The model under review builds one solid part; all positions refer to its coordinate system, in mm. Face numbers are marked on the shaded views. Round coordinates to 2 decimals unless told otherwise and drop trailing zeros. Order: outer loops, then holes, each group sorted by start corner. A loop starts at its lowest first (then second) coordinate and runs counter-clockwise, first axis right, second up. Notation, with made-up numbers: M 22,-38.75 L 58,-38.75 A8 ccw 58,-29.75 Z; hole C 83,51 d5. An arc over 180 degrees is marked long. Answer as a JSON object with one key per item and string values. Group by question number.
1. Mouldability with a two-part tool opening along X and no side actions: class the marked faces 1 and 2 as released by +X, released by -X, zero draft, split by the parting line, or undercut.
2. Add section D-D on x = 319. State the section outline as (y, z) points.
3. To check wall thickness, follow probe 1 along X at (y, z) = (-7.5, -1.5); probe 2 along X at (y, z) = (13, 0.5) (3 decimals); probe 3 along Z at (x, y) = (396, -4). State the ranges of each line that lie inside material, in increasing order. Write a range as [from, to].
4. Add section A-A on x = 400. State the section outline as (y, z) points, and give its area (3 significant figures).
5. Add section C-C on y = -6.5. State the section outline as (x, z) points.
6. Clearance check with flat-ended pins moving along their axes: P1, Ø10, axis at y = 11.5, z = 22.5, coming from the -X side; P2, Ø1, axis at x = 301.5, y = -3, coming from the -Z side; P3, Ø8, axis at y = -8.5, z = -21, coming from the +X side. State where each tip first meets the part, or that it passes through.
7. Add section B-B on z = -4. State the section outline as (x, y) points.
```python
from build123d import *

# Parameters (mm, degrees)
BOSS_EXTRUDE1_DEPTH      = 15
BOSS_EXTRUDE1_DEPTH_BACK = 15
SKETCH2_R                = 25
CUT_EXTRUDE1_DEPTH       = 30
CUT_EXTRUDE2_DEPTH       = 50


with BuildPart() as part:
    # Sketch1 → Revolve1 (revolve)
    with BuildSketch(Plane(origin=(0, 0, 0), x_dir=(1, 0, 0), z_dir=(0, 1, 0))):
        with BuildLine():
            Line((0, 11), (0, 0))
            Line((0, 0), (370, 0))
            ThreePointArc((370, 0), (370.526985697, 5.59834153), (372.089428526, 11))
            Line((372.089428526, 11), (0, 11))
        make_face()
    revolve(axis=Axis((0, 0, 0), (1, 0, 0)))

    # Sketch1_3 → Boss-Extrude1 (add, two sides: drawn at the far end of the back side and taken through both)
    with BuildSketch(Plane(origin=(0, 0, 0), x_dir=(1, 0, 0), z_dir=(0, 1, 0)).offset(-BOSS_EXTRUDE1_DEPTH_BACK)):
        with BuildLine():
            ThreePointArc((372.089428526, 11), (370.526985697, 5.59834153), (370, 0))
            Line((370, 0), (400, 0))
            Line((400, 0), (400, 11))
            Line((400, 11), (372.089428526, 11))
        make_face()
        with BuildLine():
            Line((400, 0), (370, 0))
            ThreePointArc((370, 0), (400, -30), (430, 0))
            ThreePointArc((430, 0), (405.59834153, 29.473014303), (372.089428526, 11))
            Line((372.089428526, 11), (400, 11))
            Line((400, 11), (400, 0))
        make_face()
    extrude(amount=BOSS_EXTRUDE1_DEPTH + BOSS_EXTRUDE1_DEPTH_BACK)

    # Sketch2 → Cut-Extrude1 (cut)
    with BuildSketch(Plane(origin=(0, 15, 0), x_dir=(1, 0, 0), z_dir=(0, 1, 0))):
        with Locations(Location((400, 0, 0), (0, 0, 270))):
            Circle(SKETCH2_R)
    extrude(amount=-CUT_EXTRUDE1_DEPTH, mode=Mode.SUBTRACT)

    # Sketch3 → Cut-Extrude2 (cut)
    with BuildSketch(Plane.ZY):
        with BuildLine():
            Line((-9.797958971, 5), (0, 5))
            Line((0, 5), (9.797958971, 5))
            ThreePointArc((9.797958971, 5), (0, 11), (-9.797958971, 5))
        make_face()
    extrude(amount=-CUT_EXTRUDE2_DEPTH, mode=Mode.SUBTRACT)


solid = part.part
```
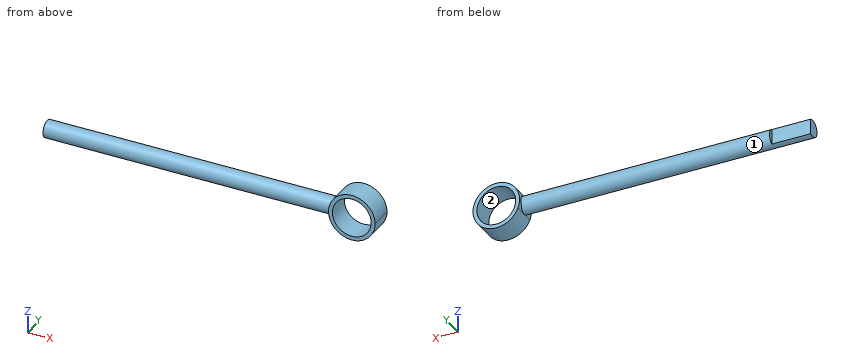
Recorded:
{
 "1": {"face 1": "zero draft", "face 2": "undercut"},
 "2": {"outline": "C 0,0 d22"},
 "3": {"probe 1": "x = [0, 375.05], [424.95, 429.96]", "probe 2": "x = [370.004, 375.005], [424.995, 429.996]", "probe 3": "z = [-29.73, -24.68], [24.68, 29.73]"},
 "4": {"outline": "M -15,-30 L 15,-30 L 15,-25 L -15,-25 Z; M -15,25 L 15,25 L 15,30 L -15,30 Z", "area": "300 mm²"},
 "5": {"outline": "M 0,-8.87 L 371.34,-8.87 A30 ccw long 371.34,8.87 L 0,8.87 Z; hole C 400,0 d50"},
 "6": {"P1": "stops at x = 375.63", "P2": "stops at z = -10.71", "P3": "stops at x = 424.72"},
 "7": {"outline": "M 0,-10.25 L 370.27,-10.25 L 370.27,-15 L 375.32,-15 L 375.32,15 L 370.27,15 L 370.27,10.25 L 50,10.25 L 50,5 L 0,5 Z; M 424.68,-15 L 429.73,-15 L 429.73,15 L 424.68,15 Z"}
}
